from build123d import *

# Parameters (mm, degrees)
ESQUISSE1_W           = 50
ESQUISSE1_H           = 10
MAIN_DEPTH            = 1
ESQUISSE2_R           = 1.5
HOLE_DEPTH            = 2
REPEATHOLERIGHT_COUNT = 3
REPEATHOLERIGHT_PITCH = 10
REPEATHOLELEFT_COUNT  = 3
REPEATHOLELEFT_PITCH  = 10


with BuildPart() as part:
    # Esquisse1 → Main (new body)
    with BuildSketch(Plane.XY):
        with Locations((25, 5)):
            Rectangle(ESQUISSE1_W, ESQUISSE1_H)
    extrude(amount=MAIN_DEPTH)

    # Esquisse2 → Hole (cut, through all)
    with BuildSketch(Plane.XY.offset(1)):
        with Locations((25, 5)):
            Circle(ESQUISSE2_R)
    hole = extrude(amount=-HOLE_DEPTH, mode=Mode.SUBTRACT)

    # RepeatHoleRight: Hole ×3
    with Locations(*[(i * REPEATHOLERIGHT_PITCH, 0, 0) for i in range(1, REPEATHOLERIGHT_COUNT)]):
        add(hole, mode=Mode.SUBTRACT)

    # RepeatHoleLeft: Hole ×3
    with Locations(*[(-i * REPEATHOLELEFT_PITCH, 0, 0) for i in range(1, REPEATHOLELEFT_COUNT)]):
        add(hole, mode=Mode.SUBTRACT)


solid = part.part
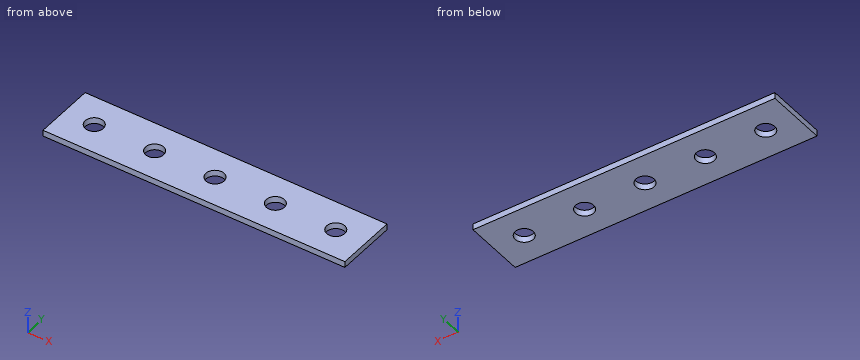
Part model, mm, in its own coordinate system. Round coordinates to 2 decimals unless told otherwise and drop trailing zeros. Loops run counter-clockwise (first coordinate to the right, second up) from the corner with the lowest first, then second, coordinate; pieces in that order, holes last. Notation, with made-up numbers: (-25, 44) - (25, 44) arc R21 cw to (25, 49) - close; hole circle Ø2 at (-16.5, 11.25). An arc over 180 degrees is marked (long way). Answer as a JSON object with one key per item and string values.
Item 1: Band-saw the part on C-C on x = 35. List the corners of the cut face in (y, z), plus the area to 3 significant figures.
Output:
{"outline": "(0, 0) - (3.5, 0) - (3.5, 1) - (0, 1) - close; (6.5, 0) - (10, 0) - (10, 1) - (6.5, 1) - close", "area": "7.00 mm2"}
Item 2: Band-saw the part on D-D on x = 14. List the corners of the cut face in (y, z).
Output:
{"outline": "(0, 0) - (3.88, 0) - (3.88, 1) - (0, 1) - close; (6.12, 0) - (10, 0) - (10, 1) - (6.12, 1) - close"}
Item 3: Band-saw the part on B-B on y = 5. List the corners of the cut face in (x, z), plus the area to 3 significant figures.
Output:
{"outline": "(0, 0) - (3.5, 0) - (3.5, 1) - (0, 1) - close; (6.5, 0) - (13.5, 0) - (13.5, 1) - (6.5, 1) - close; (16.5, 0) - (23.5, 0) - (23.5, 1) - (16.5, 1) - close; (26.5, 0) - (33.5, 0) - (33.5, 1) - (26.5, 1) - close; (36.5, 0) - (43.5, 0) - (43.5, 1) - (36.5, 1) - close; (46.5, 0) - (50, 0) - (50, 1) - (46.5, 1) - close", "area": "35.0 mm2"}
Item 4: Band-saw the part on A-A on z = 0.4. List the corners of the cut face in (x, y), plus the area to 3 significant figures.
Output:
{"outline": "(0, 0) - (50, 0) - (50, 10) - (0, 10) - close; hole circle Ø3 at (5, 5); hole circle Ø3 at (15, 5); hole circle Ø3 at (25, 5); hole circle Ø3 at (35, 5); hole circle Ø3 at (45, 5)", "area": "465 mm2"}
Item 5: Wall check: L1, parallel to Y at x = 45, z = 0.4; L2, parallel to X at y = 5.5, z = 0.7; L3, parallel to Y at x = 46, z = 0.1. Give the ranges that are in metal, low to high.
Output:
{"L1": "0 to 3.5, 6.5 to 10", "L2": "0 to 3.59, 6.41 to 13.59, 16.41 to 23.59, 26.41 to 33.59, 36.41 to 43.59, 46.41 to 50", "L3": "0 to 3.88, 6.12 to 10"}
